For this review, use the dimensioned drawing (mm, ordinates from the lowest corner) and the shaded views. A direction names the side the tool comes from. Give positions to 0.01 mm unless a question says otherwise; leave off trailing zeros. Write each loop counter-clockwise with the first axis right and the second up, starting at its lowest first coordinate (ties: lowest second). Pieces come first, ordered by that corner, then holes.
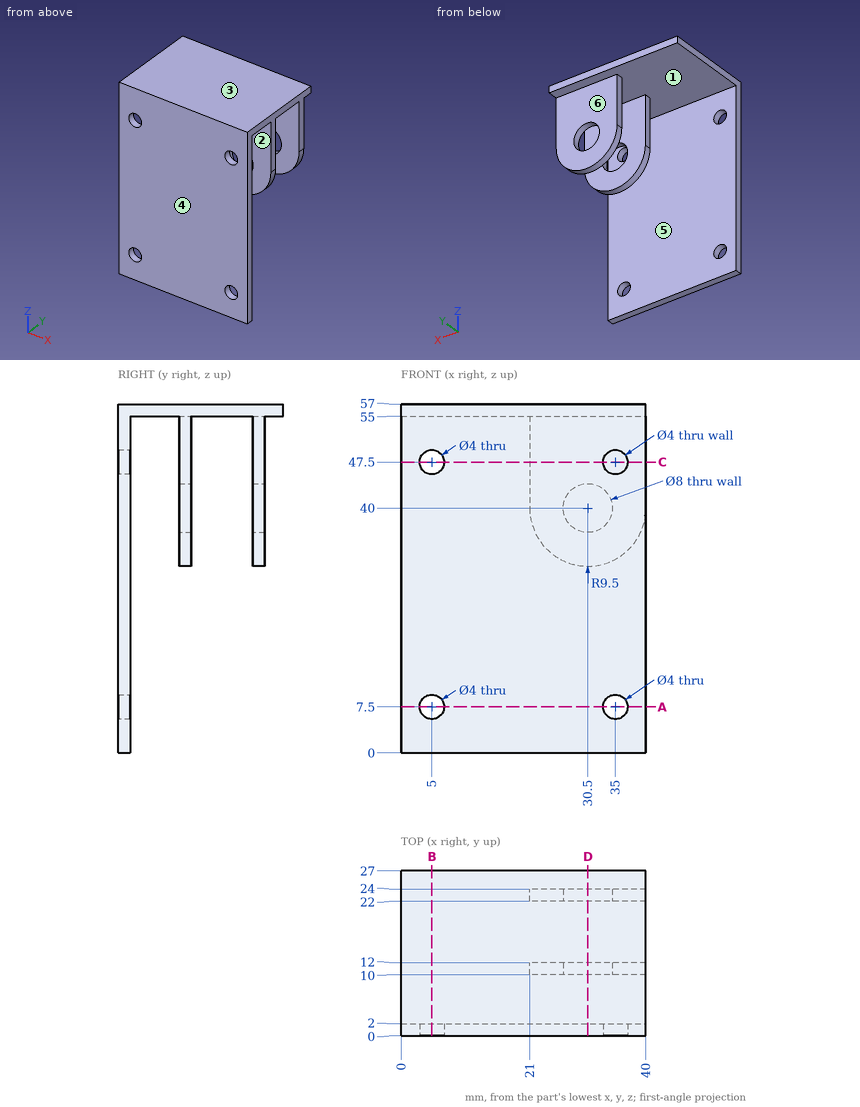
(1) We need section D-D (x = 30.5). Write out the cut boundary in (y, z).
(2) For L1, parallel to Y at x = 26, z = 50.5; L2, parallel to X at y = 1.15, z = 47.5; L3, parallel to Y at x = 34.5, z = 49, list the stretches that pass through material, from the lowest coordinate up.
(3) The part is to be moulded in two halves that separate along Y. For the marked faces 4, 5 and 6, say which applies: +Y half, -Y half, draft (parallel to the pull), parting line (faces both ways), or undercut.
(4) We need section B-B (x = 5). Write out the cut boundary in (y, z), and give its area (3 significant figures).
(5) Tool access review of the marked faces 1, 2 and 3: name each direction out of +Z, -Z, +X, -X, +Y, -Y from which nothing blocks a thin tool from reaching the whole face with its end or side.
(6) Clearance check with flat-ended pins moving along their axes: pin 1 Ø3.5 at (x, z) = (35, 47.5) entering from -Y; pin 2 Ø4.5 at (x, z) = (5, 47.5) entering from -Y; pin 3 Ø13 at (x, z) = (30.5, 40) entering from +Y; pin 4 Ø12 at (x, y) = (12, 24) entering from -Z. State where each tip first meets the part, or that it passes through.
(7) We need section C-C (z = 47.5). Write out the cut boundary in (x, y), and give its area (3 significant figures).
(8) We need section A-A (z = 7.5). Write out the cut boundary in (x, y).
The answers:
1. outline: (0, 0) - (2, 0) - (2, 55) - (10, 55) - (10, 44) - (12, 44) - (12, 55) - (22, 55) - (22, 44) - (24, 44) - (24, 55) - (27, 55) - (27, 57) - (0, 57) - close; (10, 30.5) - (12, 30.5) - (12, 36) - (10, 36) - close; (22, 30.5) - (24, 30.5) - (24, 36) - (22, 36) - close
2. L1: y = 0 to 2, 10 to 12, 22 to 24
2. L2: x = 0 to 3, 7 to 33, 37 to 40
2. L3: y = 10 to 12, 22 to 24
3. face 4: -Y half
3. face 5: undercut
3. face 6: +Y half
4. outline: (0, 0) - (2, 0) - (2, 5.5) - (0, 5.5) - close; (0, 9.5) - (2, 9.5) - (2, 45.5) - (0, 45.5) - close; (0, 49.5) - (2, 49.5) - (2, 55) - (27, 55) - (27, 57) - (0, 57) - close
4. area: 148 mm2
5. face 1: -Z, -X
5. face 2: -Z, +X, -X
5. face 3: +Z, +X, -X, +Y, -Y
6. pin 1: stops at y = 10
6. pin 2: stops at y = 0
6. pin 3: stops at y = 24
6. pin 4: stops at z = 55
7. outline: (0, 0) - (3, 0) - (3, 2) - (0, 2) - close; (7, 0) - (33, 0) - (33, 2) - (7, 2) - close; (21, 10) - (40, 10) - (40, 12) - (21, 12) - close; (21, 22) - (40, 22) - (40, 24) - (21, 24) - close; (37, 0) - (40, 0) - (40, 2) - (37, 2) - close
7. area: 140 mm2
8. outline: (0, 0) - (3, 0) - (3, 2) - (0, 2) - close; (7, 0) - (33, 0) - (33, 2) - (7, 2) - close; (37, 0) - (40, 0) - (40, 2) - (37, 2) - close
